```python
from build123d import *

# Parameters (mm, degrees)
F1_DEPTH  = 1995
F3_DEPTH  = 710
F5_DEPTH  = 1585
F7_DEPTH  = 10
F9_DEPTH  = 140
F10_R     = 10
F11_DEPTH = 25
F12_R     = 27.5
F13_DEPTH = 15
F14_R     = 27.5
F15_DEPTH = 25
F17_DEPTH = 25


with BuildPart() as f1:
    # F0 (on Right) → F1 (new body)
    with BuildSketch(Plane.YZ):
        Polygon((0, 10), (0, 0), (10, 0), (80, 0), (80, 10), (10, 10), (10, 150), (0, 150), align=None)
    extrude(amount=F1_DEPTH)

    # F2 (on face) → F3 (join)
    with BuildSketch(Plane.XZ):
        Polygon((1915, 10), (1915, 0), (1925, 0), (1995, 0), (1995, 10), (1925, 10), (1925, 150), (1915, 150), align=None)
    extrude(amount=F3_DEPTH)



with BuildPart() as f5:
    # F4 (on face) → F5 (new body)
    with BuildSketch(Plane.YZ.offset(1995)):
        Polygon((-720, 150), (-720, 10), (-790, 10), (-790, 0), (-720, 0), (-710, 0), (-710, 10), (-710, 150), align=None)
    extrude(amount=-F5_DEPTH)


with BuildPart() as f7:
    # F6 (on Top) → F7 (new body)
    with BuildSketch(Plane.XY):
        Polygon((490, -710), (80, 0), (0, 0), (410, -710), align=None)
    extrude(amount=F7_DEPTH)


with BuildPart() as f1_1:
    add(f1.part)

    add(f5.part)  # F9 merges F5

    add(f7.part)  # F9 merges F7
    # F8 (on face) → F9 (join)
    with BuildSketch(Plane.XY.offset(10)):
        Polygon((490, -710), (80, 0), (70, 0), (480, -710), align=None)
    extrude(amount=F9_DEPTH)

    # F10 (on face) → F11 (cut)
    with BuildSketch(Plane.XY.offset(10)):
        with Locations((515, -755)):
            Circle(F10_R)
        with Locations((1315, -755)):
            Circle(F10_R)
        with Locations((1793, 45)):
            Circle(F10_R)
        with Locations((193, 45)):
            Circle(F10_R)
    extrude(amount=-F11_DEPTH, mode=Mode.SUBTRACT)

    # F12 (on face) → F13 (cut)
    with BuildSketch(Plane.XZ.offset(720)):
        with Locations((445, 80)):
            Circle(F12_R)
        with Locations((1960, 80)):
            Circle(F12_R)
    extrude(amount=-F13_DEPTH, mode=Mode.SUBTRACT)

    # F14 (on face) → F15 (cut)
    with BuildSketch(Plane(origin=(0, 10, 0), x_dir=(-1, 0, 0), z_dir=(0, 1, 0))):
        with Locations((-1960, 80)):
            Circle(F14_R)
        with Locations((-35, 80)):
            Circle(F14_R)
    extrude(amount=-F15_DEPTH, mode=Mode.SUBTRACT)

    # F16 (on face) → F17 (cut)
    with BuildSketch(Plane.XY.offset(10)):
        Polygon((450.422535, -790), (410, -720), (410, -790), align=None)
    extrude(amount=-F17_DEPTH, mode=Mode.SUBTRACT)


solid = f1_1.part
```
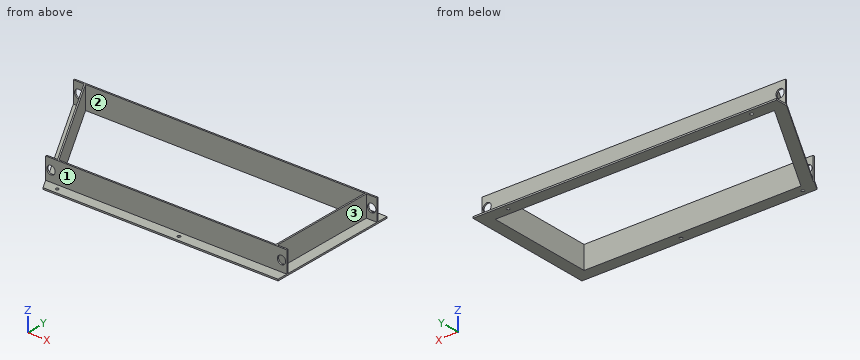
Design review of the part built by this model. Coordinates are the model's own, in mm. Face numbers are marked on the shaded views. Round coordinates to 2 decimals unless told otherwise and drop trailing zeros. Order: outer loops, then holes, each group sorted by start corner. A loop starts at its lowest first (then second) coordinate and runs counter-clockwise, first axis right, second up. Notation, with made-up numbers: (52.5, -33.5) - (107.5, -33.5) arc R11 ccw to (107.5, -27.5) - close; hole circle Ø1 at (36, -36). An arc over 180 degrees is marked (long way). Return JSON: item names as keys, results as strings.
Q1. For pin 1 Ø2 at (x, z) = (599.5, 93) entering from -Y; pin 2 Ø12 at (y, z) = (-316.5, 105) entering from +X; pin 3 Ø21 at (x, z) = (32, 53.5) entering from -Y, all flat-tipped, find the tip position at first contact; note any pin that passes through.
Computed values:
{"pin 1": "stops at y = -720", "pin 2": "stops at x = 1925", "pin 3": "stops at y = 0"}
Q2. Wall thickness on L1, parallel to Y at x = 1308.5, z = 65.5; L2, parallel to Z at x = 1960, y = -714.75; L3, parallel to X at y = -631, z = 13: over which ranges is each line inside the solid? List them lowest first. Write a range as [from, to].
Computed values:
{"L1": "y = [-720, -710], [0, 10]", "L2": "z = [0, 52.5], [107.5, 150]", "L3": "x = [434.38, 444.38], [1915, 1925]"}
Q3. Consider section B-B on y = -611.5. Write out the cut boundary in (x, z).
Computed values:
{"outline": "(353.12, 0) - (433.12, 0) - (433.12, 150) - (423.12, 150) - (423.12, 10) - (353.12, 10) - close; (1915, 0) - (1995, 0) - (1995, 10) - (1925, 10) - (1925, 150) - (1915, 150) - close"}
Q4. Consider section C-C on z = 125. Write out the cut boundary in (x, y).
Computed values:
{"outline": "(0, 0) - (70, 0) - (480, -710) - (410, -710) - (410, -720) - (1995, -720) - (1995, -710) - (1925, -710) - (1925, 0) - (1995, 0) - (1995, 10) - (0, 10) - close; hole (80, 0) - (490, -710) - (1915, -710) - (1915, 0) - close"}
Q5. Consider section A-A on x = 1835. Write out the cut boundary in (y, z).
Computed values:
{"outline": "(-790, 0) - (-710, 0) - (-710, 150) - (-720, 150) - (-720, 10) - (-790, 10) - close; (0, 0) - (80, 0) - (80, 10) - (10, 10) - (10, 150) - (0, 150) - close"}
Q6. The part is to be moulded in two halves that separate along X. For the marked faces 1, 2 and 3, say which applies: pulls with the +X half, pulls with the -X half, needs draft (parallel to the pull), parting line crosses it, or undercut.
Computed values:
{"face 1": "needs draft", "face 2": "undercut", "face 3": "pulls with the +X half"}
